```python
from build123d import *

# Parameters (mm, degrees)
ESBO_O14_W               = 40
ESBO_O14_H               = 5
RESSALTO_EXTRUS_O1_DEPTH = 3.5
ESBO_O15_W               = 30
ESBO_O15_H               = 30
ESBO_O15_R               = 1.75
RESSALTO_EXTRUS_O2_DEPTH = 5


with BuildPart() as part:
    # Esboço14 → Ressalto-extrusão1 (new, symmetric)
    with BuildSketch(Plane(origin=(0, 0, 0), x_dir=(1, 0, 0), z_dir=(0, 1, 0))):
        with Locations((-32, 0)):
            Rectangle(ESBO_O14_W, ESBO_O14_H)
    extrude(amount=RESSALTO_EXTRUS_O1_DEPTH, both=True)

    # Varredura1: sweep along a path in Esboço1
    with BuildLine(Plane.XY) as varredura1_path:
        ThreePointArc((7.070663707, 8.426488874), (-11, 0), (7.070663707, -8.426488874))
    # 3DSketch2 → Varredura1 (sweep)
    with BuildSketch(Plane(origin=(8.034845121, -9.575555539, 2.5), x_dir=(-0.33071149682512846, 0.39412661445355873, -0.8574929257125443), z_dir=(0.7660444431189768, 0.6427876096865409, 3.624573608241852e-15))):
        Polygon((0, 0), (1.543487266, 2.572478777), (5.830951895, 0), (4.287464629, -2.572478777), align=None)
    sweep(path=varredura1_path.line)

    # Esboço15 → Ressalto-extrusão2 (add)
    with BuildSketch(Plane.XY.offset(2.5)):
        with Locations((-37, 0)):
            Rectangle(ESBO_O15_W, ESBO_O15_H)
        with Locations((-48, 11)):
            Circle(ESBO_O15_R, mode=Mode.SUBTRACT)
        with Locations((-28, 11)):
            Circle(ESBO_O15_R, mode=Mode.SUBTRACT)
        with Locations((-28, -11)):
            Circle(ESBO_O15_R, mode=Mode.SUBTRACT)
        with Locations((-48, -11)):
            Circle(ESBO_O15_R, mode=Mode.SUBTRACT)
    extrude(amount=-RESSALTO_EXTRUS_O2_DEPTH)


solid = part.part
```
Verification items for the finished model (mm, model axes). A direction names the side the tool comes from. Coordinates: 2 decimals unless noted, no trailing zeros. Order: outer loops, then holes, each group sorted by start corner. A loop starts at its lowest first (then second) coordinate and runs counter-clockwise, first axis right, second up. Notation, with made-up numbers: (34.5, 2.25) -> (92.5, 2.25) arc R27 cw to (92.5, 30.25) -> close; hole circle Ø1 at (85, 72). An arc over 180 degrees is marked (long way). Answer as CSV lines item,"result". Start each with the question number.
1) Set-up check for faces 1 (the face through (-17, -3.5, 0)), 2 (the face through (7.08, 8.44, 0.03)), 3 (the face through (-29, 0, 2.5)), 4 (the face through (-37, -15, 0)), 5 (the face through (-17, 3.5, 0)): record each of +Z, -Z, +X, -X, +Y, -Y from which the full face is reachable in a straight line by a thin tool's end or side.
2) Cross-section at C-C, the plane x = 0. Record the boundary of the cut face in (y, z), then the cut area to 3 significant figures.
3) Gauge pin test, flat ends, axial feed: pin 1 Ø2 at (x, y) = (-28, 11) entering from -Z; pin 2 Ø3 at (y, z) = (11.5, 1.5) entering from +X; pin 3 Ø1.5 at (y, z) = (-11, -0.5) entering from +X; pin 4 Ø2.5 at (x, z) = (-19.5, -0.5) entering from +Y. Record the tip position at first contact, or that the pin passes through.
4) Material ranges on L1, parallel to Y at x = -48, z = 0.9; L2, parallel to X at y = -10.75, z = -1.5; L3, parallel to Y at x = -15.5, z = 0.6, recorded low to high. Write a range as [from, to].
5) Cross-section at B-B, the plane z = -0.2. Record the boundary of the cut face in (x, y).
6) Cross-section at D-D, the plane y = 11. Record the boundary of the cut face in (x, z).
7) Release check for a two-part mould opening along X. For faces 6 (the face through (-37, 15, 0)), 7 (the face through (7.08, -8.44, 0.03)), 8 (the face through (-29.75, 11.08, 0.04)), 9 (the face through (-46.331, -10.474, 0.035)) record: released by +X, released by -X, zero draft, split by the parting line, or undercut.
8) Cross-section at A-A, the plane x = -28. Record the boundary of the cut face in (y, z).
Conclusion:
1,face 1,"+Z, -Z, -Y"
1,face 2,"+Z, -Z, +X"
1,face 3,"+Z, +X, -X, +Y, -Y"
1,face 4,"+Z, -Z, +X, -X, -Y"
1,face 5,"+Z, -Z, +Y"
2,outline,"(-12.5, -2.5) -> (-9.5, -2.5) -> (-9.5, 2.5) -> (-12.5, 2.5) -> close; (9.5, -2.5) -> (12.5, -2.5) -> (12.5, 2.5) -> (9.5, 2.5) -> close"
2,area,"30.0 mm²"
3,pin 1,"passes through"
3,pin 2,"stops at x = 7.5"
3,pin 3,"stops at x = 7.15"
3,pin 4,"stops at y = 3.5"
4,L1,"y = [-15, -12.75], [-9.25, 9.25], [12.75, 15]"
4,L2,"x = [-52, -49.73], [-46.27, -29.73], [-26.27, -22], [-6.38, 6.38]"
4,L3,"y = [-3.5, 3.5]"
5,outline,"(-52, -15) -> (-22, -15) -> (-22, -3.5) -> (-12, -3.5) arc R12.5 ccw to (8.03, -9.58) -> (6.11, -7.28) arc R9.5 cw (long way) to (6.11, 7.28) -> (8.03, 9.58) arc R12.5 ccw to (-12, 3.5) -> (-22, 3.5) -> (-22, 15) -> (-52, 15) -> close; hole circle Ø3.5 at (-48, -11); hole circle Ø3.5 at (-48, 11); hole circle Ø3.5 at (-28, -11); hole circle Ø3.5 at (-28, 11)"
6,outline,"(-52, -2.5) -> (-49.75, -2.5) -> (-49.75, 2.5) -> (-52, 2.5) -> close; (-46.25, -2.5) -> (-29.75, -2.5) -> (-29.75, 2.5) -> (-46.25, 2.5) -> close; (-26.25, -2.5) -> (-22, -2.5) -> (-22, 2.5) -> (-26.25, 2.5) -> close; (-5.94, -2.5) -> (5.94, -2.5) -> (5.94, 2.5) -> (-5.94, 2.5) -> close"
7,face 6,"zero draft"
7,face 7,"released by +X"
7,face 8,"undercut"
7,face 9,"undercut"
8,outline,"(-15, -2.5) -> (-12.75, -2.5) -> (-12.75, 2.5) -> (-15, 2.5) -> close; (-9.25, -2.5) -> (9.25, -2.5) -> (9.25, 2.5) -> (-9.25, 2.5) -> close; (12.75, -2.5) -> (15, -2.5) -> (15, 2.5) -> (12.75, 2.5) -> close"
